Autodesk Inventor part; units mm, degrees
ref_plane "YZ Plane" through (0, 0, 0) normal (1, 0, 0) x (0, 1, 0)
ref_plane "XZ Plane" through (0, 0, 0) normal (0, 1, 0) x (-1, 0, 0)
ref_plane "XY Plane" through (0, 0, 0) normal (0, 0, 1) x (1, 0, 0)
sketch "Szkic1" plane through (0, 0, 0) normal (0, 1, 0) x (-1, 0, 0)
  circle A0 centre (0, 0) radius 8.5
  dimension "d0" = 17
extrude "Wyciągnięcie proste1" add sketch "Szkic1" along normal blind 57 draft 3
sketch "Szkic2" plane through (0, 57, 0) normal (0, 1, 0) x (1, 0, 0)
  circle A0 centre (0, 0) radius 11.4872
  line L0 (0, -11.4872) -> (0, 11.4872)
revolve "Obrót1" add sketch "Szkic2" angle 360 about axis through (0, 57, 11.4872) along (0, 0, -1) picked at (-4.984, 2.1752) contours L0 A0
sketch "Szkic3" plane through (0, 0, 0) normal (1, 0, 0) x (0, 1, 0)
  line L0 (0, 0) -> (0, -6.3)
  line L1 (0, -8.5) -> (0, 8.5)
  line L2 (55.7993, 11.4243) -> (55.7993, -11.4243)
  line L3 (0, 0) -> (0, 6.3)
  circle A0 centre (50, 0) radius 6.3
  line L4 (0, 6.3) -> (50, 6.3)
  line L5 (0, -6.3) -> (50, -6.3)
  point P0 (55.7993, 6.3)
  point P1 (50, 6.3)
  dimension "d4" = 6.3
  dimension "d5" = 6.3
  dimension "d13" = 50
sketch "Szkic4" plane through (0, 0, 0) normal (0, 0, 1) x (1, 0, 0)
  line L0 (0, 0) -> (5, 0)
  line L1 (8.5, 0) -> (-8.5, 0)
  line L2 (5, 0) -> (10.8623, 5.8623)
  line L3 (10.8623, 5.8623) -> (10.8623, -4.5556)
  line L4 (0, 0) -> (-5, 0)
  line L5 (-5, 0) -> (-11.3925, 6.3925)
  line L6 (-11.3925, 6.3925) -> (-11.3925, -5.0943)
  line L7 (-11.3925, -5.0943) -> (10.8623, -5.0943)
  line L8 (10.8623, -5.0943) -> (10.8623, -4.5556)
  dimension "d8" = 5
  dimension "d9" = 135
  dimension "d10" = 5
extrude "Wyciągnięcie proste3" cut sketch "Szkic4" along normal mid plane 30
extrude "Wyciągnięcie proste4" cut sketch "Szkic3" along normal mid plane 6
properties material "Kauczuk"
Geometry check sheet. Reference: the model listing, model coordinates, mm. A direction names the side the tool comes from. Coordinates: 2 decimals unless noted, no trailing zeros. Order: outer loops, then holes, each group sorted by start corner. A loop starts at its lowest first (then second) coordinate and runs counter-clockwise, first axis right, second up. Notation, with made-up numbers: (48.5, 5.5) -> (53.5, 5.5) arc R28 cw to (53.5, 28.5) -> close; hole circle Ø1 at (-24, -27). An arc over 180 degrees is marked (long way). Use a Markdown table: item, result. Add a question column.
1. Mould release check, pull along Z, two halves, no side actions. Record for faces 3 (the face through (-3, 28, 0)), 4 (the face through (3.4, 0, 0.1)), 5 (the face through (-9.221, 28.291, -3.823)): pulls with the +Z half, pulls with the -Z half, needs draft (parallel to the pull), parting line crosses it, or undercut.
2. Set-up check for faces 1 (the face through (6, 1, 0)), 2 (the face through (0, 25, -6.3)): record each of +Z, -Z, +X, -X, +Y, -Y from which the full face is reachable in a straight line by a thin tool's end or side.
3. Go/stop test with flat-tipped pins: pin 1 Ø5 at (x, y) = (1.5, 32.5) entering from +Z; pin 2 Ø1 at (x, y) = (-8, 29.5) entering from -Z; pin 3 Ø4 at (x, y) = (-1.5, 26.5) entering from +Z. Record where each tip stops, or that it passes through.
4. Cross-section at C-C (y = 22.5). Enter the section's corners in (x, z), and give its area (3 significant figures).
5. Cross-section at B-B (y = 7.5). Enter the section's corners in (x, z), and give its area (3 significant figures).
6. Material ranges on L1, parallel to X at y = 37, z = 6; L2, parallel to X at y = 26, z = 3.25; L3, parallel to X at y = 64.5, z = 0, recorded low to high.
Filled sheet:
| question | item | result |
|---|---|---|
| 1 | face 3 | undercut |
| 1 | face 4 | needs draft |
| 1 | face 5 | parting line crosses it |
| 2 | face 1 | +Z, -Z, +X, -Y |
| 2 | face 2 | -Y |
| 3 | pin 1 | z = 10.31 |
| 3 | pin 2 | z = -6.69 |
| 3 | pin 3 | z = 9.97 |
| 4 | outline | circle Ø19.36 at (0, 0); hole (-3, -6.3) -> (3, -6.3) -> (3, 6.3) -> (-3, 6.3) -> close |
| 4 | area | 219 mm2 |
| 5 | outline | circle Ø17.79 at (0, 0); hole (-3, -6.3) -> (3, -6.3) -> (3, 6.3) -> (-3, 6.3) -> close |
| 5 | area | 173 mm2 |
| 6 | L1 | -8.54 to -3, 3 to 8.54 |
| 6 | L2 | -9.31 to -3, 3 to 9.31 |
| 6 | L3 | -8.7 to 8.7 |
